For this review, use the dimensioned drawing (mm, ordinates from the lowest corner) and the shaded views. Give positions to 0.01 mm unless a question says otherwise; leave off trailing zeros. Order: outer loops, then holes, each group sorted by start corner. A loop starts at its lowest first (then second) coordinate and runs counter-clockwise, first axis right, second up. Notation, with made-up numbers: (44.5, 24) - (82.5, 24) arc R22 ccw to (82.5, 55) - close; hole circle Ø3 at (72, 81). An arc over 180 degrees is marked (long way). One line per item, written item: value.
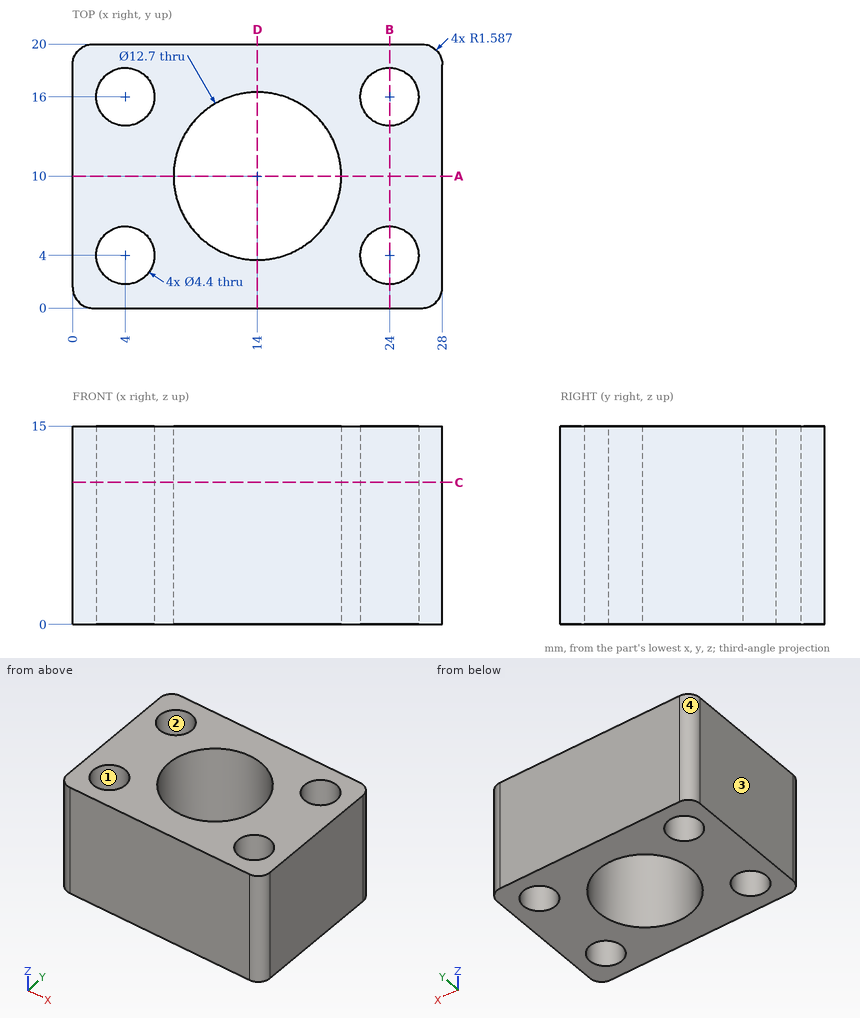
(1) Wall thickness on line 1 (Y direction, x = 24, z = 11); line 2 (Y direction, x = 14, z = 5); line 3 (Y direction, x = 24.5, z = 2.25): over which ranges is each line inside the solid? List them lowest first. Write a range as from..to.
Answers below:
line 1: y = 0..1.8, 6.2..13.8, 18.2..20
line 2: y = 0..3.65, 16.35..20
line 3: y = 0..1.86, 6.14..13.86, 18.14..20
(2) Take a section at C-C (z = 10.75). Give the number of separate pieces and of enclosed holes in the cut face.
Answers below:
separate pieces: 1
enclosed holes: 5
(3) Take a section at B-B (x = 24). Write out the cut boundary in (y, z), then the cut area to 3 significant figures.
Answers below:
outline: (0, 0) - (1.8, 0) - (1.8, 15) - (0, 15) - close; (6.2, 0) - (13.8, 0) - (13.8, 15) - (6.2, 15) - close; (18.2, 0) - (20, 0) - (20, 15) - (18.2, 15) - close
area: 168 mm^2
(4) Take a section at D-D (x = 14). Write out the cut boundary in (y, z).
Answers below:
outline: (0, 0) - (3.65, 0) - (3.65, 15) - (0, 15) - close; (16.35, 0) - (20, 0) - (20, 15) - (16.35, 15) - close
(5) Draft analysis for pull direction Y (two halves, no side actions). For the marked faces 1, 2, 3 and 4, state which applies: pulls with the +Y half, pulls with the -Y half, needs draft (parallel to the pull), parting line crosses it, or undercut.
Answers below:
face 1: undercut
face 2: undercut
face 3: needs draft
face 4: pulls with the +Y half
(6) For P1, Ø4, axis at x = 4, y = 16, coming from the +Z side, flat-tipped, find the tip position at first contact; note if it passes through.
Answers below:
P1: passes through
(7) Take a section at A-A (y = 10). Write out the cut boundary in (x, z).
Answers below:
outline: (0, 0) - (7.65, 0) - (7.65, 15) - (0, 15) - close; (20.35, 0) - (28, 0) - (28, 15) - (20.35, 15) - close
